```python
from build123d import *

# Parameters (mm, degrees)
SKETCH_1_W          = 20
SKETCH_1_H          = 35
EXTRUDE_1_DEPTH     = 5
SKETCH_2_W          = 10
SKETCH_2_H          = 14.8
EXTRUDE_2_DEPTH     = 10
SKETCH_3_W          = 20
SKETCH_3_H          = 35
EXTRUDE_3_DEPTH     = 5
SKETCH_4_R          = 1
CUT_EXTRUDE_1_DEPTH = 34.260336739
SKETCH_5_R          = 1.5
CUT_EXTRUDE_2_DEPTH = 29.394541729
SKETCH_6_W          = 11.5
SKETCH_6_H          = 14.8
CUT_EXTRUDE_3_DEPTH = 10


with BuildPart() as part:
    # ｽｹｯﾁ1 → ﾎﾞｽ - 押し出し1 (new body)
    with BuildSketch(Plane.XY):
        Rectangle(SKETCH_1_W, SKETCH_1_H)
    extrude(amount=EXTRUDE_1_DEPTH)

    # ｽｹｯﾁ2 → ﾎﾞｽ - 押し出し2 (add)
    with BuildSketch(Plane.XY.offset(5)):
        with Locations((5, -10.1)):
            Rectangle(SKETCH_2_W, SKETCH_2_H)
    extrude(amount=EXTRUDE_2_DEPTH)

    # ｽｹｯﾁ3 → ﾎﾞｽ - 押し出し3 (add)
    with BuildSketch(Plane.XY.offset(15)):
        Rectangle(SKETCH_3_W, SKETCH_3_H)
    extrude(amount=EXTRUDE_3_DEPTH)

    # ｽｹｯﾁ4 → ｶｯﾄ - 押し出し1 (cut, through all)
    with BuildSketch(Plane(origin=(10, 0, 0), x_dir=(0, 0, -1), z_dir=(1, 0, 0))):
        with Locations((-15, -2.7)):
            Circle(SKETCH_4_R)
        with Locations((-5, -2.7)):
            Circle(SKETCH_4_R)
    extrude(amount=-CUT_EXTRUDE_1_DEPTH, mode=Mode.SUBTRACT)

    # ｽｹｯﾁ5 → ｶｯﾄ - 押し出し2 (cut, through all)
    with BuildSketch(Plane.XY.offset(20)):
        with Locations((0, 12.5)):
            Circle(SKETCH_5_R)
        with Locations((0, 2.5)):
            Circle(SKETCH_5_R)
    extrude(amount=-CUT_EXTRUDE_2_DEPTH, mode=Mode.SUBTRACT)

    # ｽｹｯﾁ6 → ｶｯﾄ - 押し出し3 (cut)
    with BuildSketch(Plane.ZY):
        with Locations((10, -10.1)):
            Rectangle(SKETCH_6_W, SKETCH_6_H)
    extrude(amount=CUT_EXTRUDE_3_DEPTH, mode=Mode.SUBTRACT)


solid = part.part
```
Source: CAD feature listing. Evaluate the final solid. Frame: model axes, mm. A direction names the side the tool comes from. Round coordinates to 2 decimals unless told otherwise and drop trailing zeros. Loops run counter-clockwise (first coordinate to the right, second up) from the corner with the lowest first, then second, coordinate; pieces in that order, holes last. Notation, with made-up numbers: M 27.5,27.5 L 31.5,27.5 A17 cw 31.5,40.5 Z; hole C 79,81.5 d5. An arc over 180 degrees is marked long. Use a Markdown table: item, result. Add a question column.
1. Section query C-C on z = 3. Return the cut outline in (x, y).
2. Contact query for flat-ended pins moving along their axis: P1, Ø3.5, axis at x = 0, y = 2.5, coming from the -Z side; P2, Ø9, axis at x = 7.5, z = 10, coming from the +Y side. Output: stop coordinate, or through.
3. Mould query, pull axis X, two halves, no side actions, for faces 1 (the cylindrical face through (0, 1, 18)), 2 (the flat face through (0, -10, 10)), 3 (the flat face through (0, 8, 5)), 4 (the cylindrical face through (0, 11, 3)). Classes: pulls with the +X half, pulls with the -X half, needs draft (parallel to the pull), parting line crosses it, or undercut.
4. Section query D-D on y = -13. Return the cut outline in (x, z).
5. Line query: line 1 (Y direction, x = 0, z = 16.2); line 2 (Z direction, x = 6.5, y = 2.5); line 3 (Z direction, x = -4.5, y = -14.5). Output: solid intervals per line, ascending.
6. Section query B-B on x = -6.75. Return the cut outline in (y, z).
7. Section query A-A on y = 12.5. Return the cut outline in (x, z), then the cut area to 3 significant figures.
8. Reachability of faces 5 (the flat face through (0, 8, 15)), 6 (the flat face through (-5, -11, 15.75)), 7 (the flat face through (0, 17.5, 17)) from +Z, -Z, +X, -X, +Y, -Y: full face, straight path, thin tool, end or side. Return the list, or none.
Reported:
| question | item | result |
|---|---|---|
| 1 | outline | M -10,-17.5 L 10,-17.5 L 10,17.5 L -10,17.5 Z; hole C 0,2.5 d3; hole C 0,12.5 d3 |
| 2 | P1 | stops at z = 0 |
| 2 | P2 | stops at y = -2.7 |
| 3 | face 1 | undercut |
| 3 | face 2 | pulls with the -X half |
| 3 | face 3 | needs draft |
| 3 | face 4 | undercut |
| 4 | outline | M -10,0 L 10,0 L 10,20 L -10,20 L -10,15.75 L 0,15.75 L 0,4.25 L -10,4.25 Z |
| 5 | line 1 | y = -17.5 to 1, 4 to 11, 14 to 17.5 |
| 5 | line 2 | z = 0 to 5, 15 to 20 |
| 5 | line 3 | z = 0 to 4.25, 15.75 to 20 |
| 6 | outline | M -17.5,0 L 17.5,0 L 17.5,5 L -1.7,5 A1 cw -3.36,4.25 L -17.5,4.25 Z; M -17.5,15.75 L -3.36,15.75 A1 cw -1.7,15 L 17.5,15 L 17.5,20 L -17.5,20 Z |
| 7 | outline | M -10,0 L -1.5,0 L -1.5,5 L -10,5 Z; M -10,15 L -1.5,15 L -1.5,20 L -10,20 Z; M 1.5,0 L 10,0 L 10,5 L 1.5,5 Z; M 1.5,15 L 10,15 L 10,20 L 1.5,20 Z |
| 7 | area | 170 mm² |
| 8 | face 5 | +X, -X, +Y |
| 8 | face 6 | -X, -Y |
| 8 | face 7 | +Z, -Z, +X, -X, +Y |
